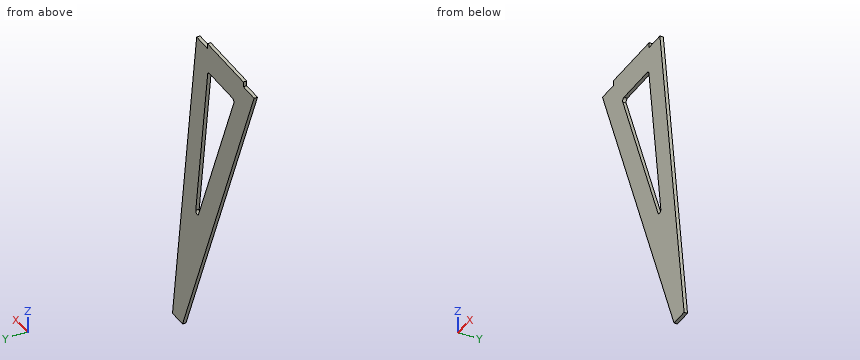
```python
from build123d import *

# Parameters (mm, degrees)
BOSS_EXTRUDE1_DEPTH = 3.175
CUT_EXTRUDE1_REACH  = 336.078
FILLET1_R           = 2.54
SKETCH3_W           = 63.5
SKETCH3_H           = 3.175
BOSS_EXTRUDE2_DEPTH = 4.7625


with BuildPart() as part:
    # Sketch1 → Boss-Extrude1 (new body)
    with BuildSketch(Plane(origin=(0, 0, 0), x_dir=(1, 0, 0), z_dir=(0, 1, 0))):
        Polygon((0, 301.244), (-42.794923706, 0), (-144.394923706, 0), (-17.78, 301.244), align=None)
    extrude(amount=BOSS_EXTRUDE1_DEPTH)

    # Sketch2 → Cut-Extrude1 (cut, up to next)
    with BuildSketch(Plane(origin=(0, 3.175, 0), x_dir=(1, 0, 0), z_dir=(0, 1, 0)), mode=Mode.PRIVATE) as cut_extrude1_sk1:
        Polygon((-38.460690081, 193.042545844), (-109.989583795, 22.86), (-62.636936132, 22.86), align=None)
    cut_extrude1_tool1 = extrude(cut_extrude1_sk1.sketch, amount=-CUT_EXTRUDE1_REACH, mode=Mode.PRIVATE) & part.part
    add(cut_extrude1_tool1.solids().sort_by_distance((-70.362403, 3.175, -79.587515))[0], mode=Mode.SUBTRACT)

    # Fillet1
    fillet1_edges = [part.edges().sort_by_distance(p)[0] for p in [
        (-38.460690081, 1.5875, -193.042545844),
        (-62.636936132, 1.5875, -22.86),
        (-109.989583795, 1.5875, -22.86),
    ]]
    fillet(fillet1_edges, radius=FILLET1_R)

    # Sketch3 → Boss-Extrude2 (add)
    with BuildSketch(Plane.XY):
        with Locations((-93.594923706, 1.5875)):
            Rectangle(SKETCH3_W, SKETCH3_H)
    extrude(amount=BOSS_EXTRUDE2_DEPTH)


solid = part.part
```
Here's how the part is built. I have some questions about the finished solid (model axes, mm). Give positions to 0.01 mm unless a question says otherwise; leave off trailing zeros. Order: outer loops, then holes, each group sorted by start corner. A loop starts at its lowest first (then second) coordinate and runs counter-clockwise, first axis right, second up. Notation, with made-up numbers: (18, 86) - (71, 86) arc R17 ccw to (71, 94) - close; hole circle Ø2 at (-24, 5.5). An arc over 180 degrees is marked (long way). Answer as a JSON object with one key per item and string values. Group by question number.
Item 1: If we section it at D-D on x = -135: Please give me the cut outline in (y, z) (3 decimals), and give its area (3 significant figures).
Item 2: If we section it at B-B on x = -68: Please give me the cut outline in (y, z) (1 decimal).
Item 3: If we section it at C-C on z = -31: Please give me the cut outline in (x, y) (3 decimals).
Item 4: For P1, Ø1, axis at x = -55.5, y = 1, coming from the +Z side, with a flat end and sliding along its axis, tell me the tip position at first contact or that it passes through.
Item 5: Please list where these lines run through material, in increasing order: probe 1 along X at (y, z) = (1.5, -29.5); probe 2 along X at (y, z) = (2.8, -88); probe 3 along Z at (x, y) = (-66.5, 0.85).
Item 6: If we section it at A-A on y = 1.85: Please give me the cut outline in (x, z).
Result set:
{
 "1": {"outline": "(0, -22.353) - (3.175, -22.353) - (3.175, 0) - (0, 0) - close", "area": "71.0 mm²"},
 "2": {"outline": "(0, -181.8) - (3.2, -181.8) - (3.2, -122.8) - (0, -122.8) - close; (0, -22.9) - (3.2, -22.9) - (3.2, 4.8) - (0, 4.8) - close"},
 "3": {"outline": "(-131.365, 0) - (-106.568, 0) - (-106.568, 3.175) - (-131.365, 3.175) - close; (-61.481, 0) - (-38.391, 0) - (-38.391, 3.175) - (-61.481, 3.175) - close"},
 "4": {"P1": "z = 0"},
 "5": {"probe 1": "-132 to -107.2, -61.69 to -38.6", "probe 2": "-107.41 to -82.61, -53.38 to -30.29", "probe 3": "-185.33 to -126.33, -22.86 to 4.76"},
 "6": {"outline": "(-144.39, 0) - (-17.78, -301.24) - (0, -301.24) - (-42.79, 0) - (-61.84, 0) - (-61.84, 4.76) - (-125.34, 4.76) - (-125.34, 0) - close; hole (-108.51, -26.38) - (-46.08, -174.9) arc R2.54 ccw to (-41.23, -173.56) - (-62.33, -25.04) arc R2.54 ccw to (-64.84, -22.86) - (-106.17, -22.86) arc R2.54 ccw to start"}
}
